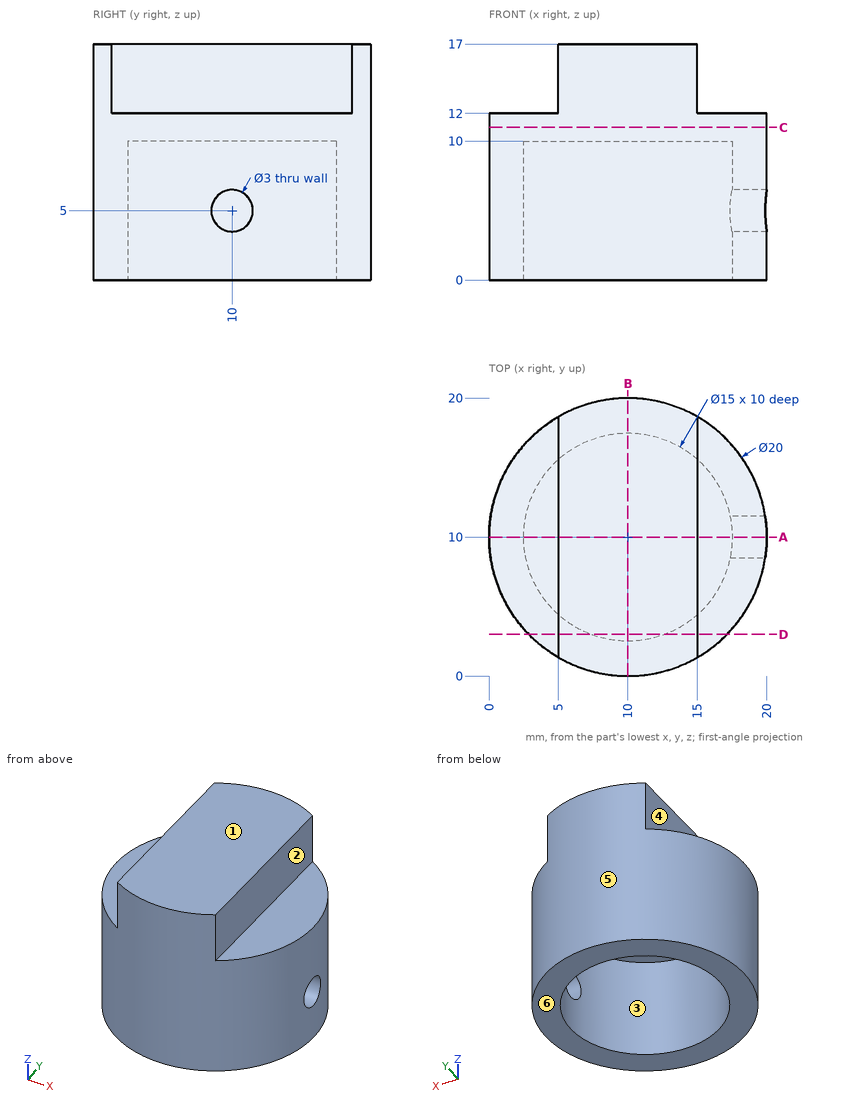
The drawing under review shows one solid part. Ordinate dimensions are in mm from its lowest x, y, z. A direction names the side the tool comes from. Round coordinates to 2 decimals unless told otherwise and drop trailing zeros. Loops run counter-clockwise (first coordinate to the right, second up) from the corner with the lowest first, then second, coordinate; pieces in that order, holes last. Notation, with made-up numbers: (68.5, 57.25) - (91.5, 57.25) arc R33 ccw to (91.5, 88.25) - close; hole circle Ø1 at (-39, 63.25). An arc over 180 degrees is marked (long way). One line per question, with ' | ' between items.
1. For L1, parallel to Y at x = 10, z = 3.75; L2, parallel to Y at x = 13.5, z = 2; L3, parallel to X at y = 12.75, z = 7, list the stretches that pass through material, from the lowest coordinate up. Write a range as [from, to].
Results are:
L1: y = [0, 2.5], [17.5, 20] | L2: y = [0.63, 3.37], [16.63, 19.37] | L3: x = [0.39, 3.02], [16.98, 19.61]
2. Draft analysis for pull direction X (two halves, no side actions). For the marked faces 3, 4, 5 and 6, state which applies: released by +X, released by -X, zero draft, split by the parting line, or undercut.
Results are:
face 3: undercut | face 4: released by -X | face 5: split by the parting line | face 6: zero draft
3. We need section A-A, the plane y = 10. State the section outline as (x, z) points.
Results are:
outline: (0, 0) - (2.5, 0) - (2.5, 10) - (17.5, 10) - (17.5, 6.5) - (20, 6.5) - (20, 12) - (15, 12) - (15, 17) - (5, 17) - (5, 12) - (0, 12) - close; (17.5, 0) - (20, 0) - (20, 3.5) - (17.5, 3.5) - close
4. We need section C-C, the plane z = 11. State the section outline as (x, y) points.
Results are:
outline: circle Ø20 at (10, 10)
5. Clearance check with flat-ended pins moving along their axes: P1, Ø4, axis at x = 13, y = 8.5, coming from the -Z side; P2, Ø2.5, axis at x = 18, y = 11, coming from the +Z side; P3, Ø1.5, axis at y = 11.5, z = 14.5, coming from the +X side. State where each tip first meets the part, or that it passes through.
Results are:
P1: stops at z = 10 | P2: stops at z = 12 | P3: stops at x = 15
6. We need section B-B, the plane x = 10. State the section outline as (y, z) points.
Results are:
outline: (0, 0) - (2.5, 0) - (2.5, 10) - (17.5, 10) - (17.5, 0) - (20, 0) - (20, 17) - (0, 17) - close
7. For the marked faces 1 and 2, list the 3-axis set-ups (+Z, -Z, +X, -X, +Y, -Y) from which the entire face can be reached by the end or side of a thin tool; tool diameter is ignored.
Results are:
face 1: +Z, +X, -X, +Y, -Y | face 2: +Z, +X, +Y, -Y
8. We need section D-D, the plane y = 3. State the section outline as (x, z) points, and give its area (3 significant figures).
Results are:
outline: (2.86, 0) - (7.31, 0) - (7.31, 10) - (12.69, 10) - (12.69, 0) - (17.14, 0) - (17.14, 12) - (15, 12) - (15, 17) - (5, 17) - (5, 12) - (2.86, 12) - close | area: 168 mm²
